For this review, take the finished solid that the model builds, in its own axes (mm). Round coordinates to 2 decimals unless told otherwise and drop trailing zeros. Write each loop counter-clockwise with the first axis right and the second up, starting at its lowest first coordinate (ties: lowest second). Pieces come first, ordered by that corner, then holes. Notation, with made-up numbers: (7, 38) - (37, 38) arc R15 ccw to (37, 61) - close; hole circle Ø5 at (-16.5, 84.25). An arc over 180 degrees is marked (long way). Answer in a Markdown table with one row per item. Add a question column.
from build123d import *

# Parameters (mm, degrees)
BOSS_EXTRUDE1_DEPTH = 6


with BuildPart() as part:
    # Sketch1 → Boss-Extrude1 (new body)
    with BuildSketch(Plane.XY):
        with BuildLine():
            Line((-149, -191.5), (-149, -197.5))
            Line((-149, -197.5), (-50.5, -197.5))
            Line((-50.5, -197.5), (-50.5, -167.5))
            ThreePointArc((-50.5, -167.5), (0, -117), (50.5, -167.5))
            Line((50.5, -167.5), (50.5, -191.5))
            Line((50.5, -191.5), (191.5, -191.5))
            Line((191.5, -191.5), (191.5, -96.5))
            Line((191.5, -96.5), (197.5, -96.5))
            Line((197.5, -96.5), (197.5, 0))
            Line((197.5, 0), (191.5, 0))
            Line((191.5, 0), (191.5, 101))
            Line((191.5, 101), (197.5, 101))
            Line((197.5, 101), (197.5, 197.5))
            Line((197.5, 197.5), (-191.5, 197.5))
            Line((-191.5, 197.5), (-191.5, 96.5))
            Line((-191.5, 96.5), (-197.5, 96.5))
            Line((-197.5, 96.5), (-197.5, 0))
            Line((-197.5, 0), (-191.5, 0))
            Line((-191.5, 0), (-191.5, -101))
            Line((-191.5, -101), (-197.5, -101))
            Line((-197.5, -101), (-197.5, -191.5))
            Line((-197.5, -191.5), (-149, -191.5))
        make_face()
    extrude(amount=BOSS_EXTRUDE1_DEPTH)


solid = part.part
Q1. Draft analysis for pull direction X (two halves, no side actions). For faces 1 (the face through (-1.11, -117.012, 2.958)), 2 (the face through (-3, 3, 0)), state which applies: released by +X, released by -X, zero draft, split by the parting line, or undercut.
Q2. Insertion check: pin 1 Ø2 at (y, z) = (-101.5, 2.5) entering from +X; pin 2 Ø1.8 at (x, z) = (195.5, 3.5) entering from -Y; pin 3 Ø3 at (y, z) = (-28, 1.5) entering from -X. Each pin has a flat end and moves straight along its axis. Give the tip position at first contact, or say it passes through.
Q3. Add section A-A on y = -145.5. State the section outline as (x, z) points, then the cut area to 3 significant figures.
Q4. Add section B-B on z = 3.15. State the section outline as (x, y) points, then the cut area to 3 significant figures.
Q5. To check wall thickness, follow probe 1 along Y at (x, z) = (72, 3.05); probe 2 along X at (y, z) = (15, 3.55). State the ranges of each line that lie inside material, in increasing order.
Q6. Add section D-D on y = 84. State the section outline as (x, z) points, then the cut area to 3 significant figures.
Q7. Add section C-C on x = -155.5. State the section outline as (y, z) points, then the cut area to 3 significant figures.
Answer sheet:
| question | item | result |
|---|---|---|
| 1 | face 1 | undercut |
| 1 | face 2 | zero draft |
| 2 | pin 1 | stops at x = 191.5 |
| 2 | pin 2 | stops at y = -96.5 |
| 2 | pin 3 | stops at x = -191.5 |
| 3 | outline | (-197.5, 0) - (-45.46, 0) - (-45.46, 6) - (-197.5, 6) - close; (45.46, 0) - (191.5, 0) - (191.5, 6) - (45.46, 6) - close |
| 3 | area | 1,790 mm² |
| 4 | outline | (-197.5, -191.5) - (-149, -191.5) - (-149, -197.5) - (-50.5, -197.5) - (-50.5, -167.5) arc R50.5 cw to (50.5, -167.5) - (50.5, -191.5) - (191.5, -191.5) - (191.5, -96.5) - (197.5, -96.5) - (197.5, 0) - (191.5, 0) - (191.5, 101) - (197.5, 101) - (197.5, 197.5) - (-191.5, 197.5) - (-191.5, 96.5) - (-197.5, 96.5) - (-197.5, 0) - (-191.5, 0) - (-191.5, -101) - (-197.5, -101) - close |
| 4 | area | 145,000 mm² |
| 5 | probe 1 | y = -191.5 to 197.5 |
| 5 | probe 2 | x = -197.5 to 191.5 |
| 6 | outline | (-197.5, 0) - (191.5, 0) - (191.5, 6) - (-197.5, 6) - close |
| 6 | area | 2,330 mm² |
| 7 | outline | (-191.5, 0) - (197.5, 0) - (197.5, 6) - (-191.5, 6) - close |
| 7 | area | 2,330 mm² |
